```python
from build123d import *

# Parameters (mm, degrees)
F1_DEPTH = 457.2


with BuildPart() as f1:
    # F0 (on Front) → F1 (new body, symmetric)
    with BuildSketch(Plane.XZ):
        with BuildLine():
            Line((-1219.2, 0), (-2.630256, 0))
            ThreePointArc((-2.630256, 0), (-0.200216, 0.483365), (1.859872, 1.859872))
            Line((1.859872, 1.859872), (302.940128, 302.940128))
            ThreePointArc((302.940128, 302.940128), (305.000216, 304.316635), (307.430256, 304.8))
            Line((307.430256, 304.8), (1219.2, 304.8))
            Line((1219.2, 304.8), (1219.2, 311.15))
            Line((1219.2, 311.15), (304.8, 311.15))
            ThreePointArc((304.8, 311.15), (302.36996, 310.666635), (300.309872, 309.290128))
            Line((300.309872, 309.290128), (-0.770384, 8.209872))
            ThreePointArc((-0.770384, 8.209872), (-2.830472, 6.833365), (-5.260512, 6.35))
            Line((-5.260512, 6.35), (-1219.2, 6.35))
            Line((-1219.2, 6.35), (-1219.2, 0))
        make_face()
    extrude(amount=F1_DEPTH, both=True)


solid = f1.part
```
The listing builds one solid part. Answer for the finished solid, in the listing's coordinates (mm). A direction names the side the tool comes from. Give positions to 0.01 mm unless a question says otherwise; leave off trailing zeros. Order: outer loops, then holes, each group sorted by start corner. A loop starts at its lowest first (then second) coordinate and runs counter-clockwise, first axis right, second up. Notation, with made-up numbers: (75, 67.25) -> (116, 67.25) arc R10 cw to (116, 72.25) -> close; hole circle Ø8 at (80.5, 19). An arc over 180 degrees is marked (long way). One line per item, written item: value.
1) Find section B-B, the plane x = -76. Determine the outline of the cut face in (y, z).
Reported:
outline: (-457.2, 0) -> (457.2, 0) -> (457.2, 6.35) -> (-457.2, 6.35) -> close
2) Flat-ended cylindrical pins translate along their axes: P1, Ø4, axis at y = -251.5, z = 205, coming from the -X side; P2, Ø12, axis at y = 24, z = 200, coming from the -X side; P3, Ø8, axis at y = -280, z = 131.5, coming from the -X side. Find the tip coordinate at first contact, or state that the pin passes through.
Reported:
P1: stops at x = 194.02
P2: stops at x = 185.02
P3: stops at x = 118.52
3) A tool of negligible diameter and unlimited length cuts with its end or side. For faces 1 (the flat face through (-619, -6, 0)), 2 (the flat face through (757, -6, 304.8)), 3 (the flat face through (-604, -6, 6.35)), from which of +Z, -Z, +X, -X, +Y, -Y can it reach the whole face along a straight path? Write none if from no direction.
Reported:
face 1: -Z, +X, -X, +Y, -Y
face 2: -Z, +X, +Y, -Y
face 3: +Z, -X, +Y, -Y
4) Find the intervals of material crossed by line 1 (Z direction, x = -361.5, y = 376); line 2 (Z direction, x = 1023.5, y = 284.5); line 3 (X direction, y = 338, z = 244.5), in increasing order.
Reported:
line 1: z = 0 to 6.35
line 2: z = 304.8 to 311.15
line 3: x = 235.52 to 244.5
5) Find section A-A, the plane y = 98.5. Determine the outline of the cut face in (x, z).
Reported:
outline: (-1219.2, 0) -> (-2.63, 0) arc R6.35 ccw to (1.86, 1.86) -> (302.94, 302.94) arc R6.35 cw to (307.43, 304.8) -> (1219.2, 304.8) -> (1219.2, 311.15) -> (304.8, 311.15) arc R6.35 ccw to (300.31, 309.29) -> (-0.77, 8.21) arc R6.35 cw to (-5.26, 6.35) -> (-1219.2, 6.35) -> close
6) Find section C-C, the plane z = 31. Determine the outline of the cut face in (x, y).
Reported:
outline: (22.02, -457.2) -> (31, -457.2) -> (31, 457.2) -> (22.02, 457.2) -> close
